Can you work these out from the model? Positions are in its coordinate system, mm. A direction names the side the tool comes from. Give positions to 0.01 mm unless a question says otherwise; leave off trailing zeros. Order: outer loops, then holes, each group sorted by start corner. A loop starts at its lowest first (then second) coordinate and runs counter-clockwise, first axis right, second up. Notation, with made-up numbers: (26, 27) - (55, 27) arc R23 cw to (55, 60) - close; hole circle Ø9 at (53.5, 45.25). An arc over 180 degrees is marked (long way). Answer as a JSON object with one key per item and string values.
```python
from build123d import *

# Parameters (mm, degrees)
F0_W       = 43.8023
F0_H       = 40.5003
F0_R       = 9.72185
F1_DEPTH   = 9.0424
F3_DEPTH   = 25.4
F4_SIZE2   = 2.54
F4_SIZE    = 0.762
F4_2_SIZE2 = 2.54
F4_2_SIZE  = 0.762
F5_R       = 12.65555
F6_DEPTH   = 2.667
F7_R       = 0.254


with BuildPart() as f1:
    # F0 (on Front) → F1 (new body)
    with BuildSketch(Plane.XZ):
        Rectangle(F0_W, F0_H)
        Circle(F0_R, mode=Mode.SUBTRACT)
    extrude(amount=F1_DEPTH)

    # F2 (on Top) → F3 (cut, symmetric)
    with BuildSketch(Plane.XY):
        Polygon((17.653, -6.096), (17.653, -9.144), (17.653, -9.8752817139), (22.691456601, -9.8752817139), (22.691456601, -6.096), align=None)
        Polygon((-17.653, -9.8752817139), (-17.653, -9.144), (-17.653, -6.096), (-22.691456601, -6.096), (-22.691456601, -9.8752817139), align=None)
    extrude(amount=F3_DEPTH, both=True, mode=Mode.SUBTRACT)

    # F4
    f4_edges = [f1.edges().sort_by_distance(p)[0] for p in [
        (-21.90115, 0, 0),
    ]]
    f4_side = f1.faces().sort_by_distance((-21.90115, -3.048, 0))[0]
    chamfer(f4_edges, length=F4_SIZE, length2=F4_SIZE2, reference=f4_side)

    # F4#2
    f4_2_edges = [f1.edges().sort_by_distance(p)[0] for p in [
        (21.90115, 0, 0),
    ]]
    f4_2_side = f1.faces().sort_by_distance((21.90115, -3.048, 0))[0]
    chamfer(f4_2_edges, length=F4_2_SIZE, length2=F4_2_SIZE2, reference=f4_2_side)

    # F5 (on face) → F6 (cut)
    with BuildSketch(Plane(origin=(0, 0, 0), x_dir=(-1, 0, 0), z_dir=(0, 1, 0))):
        Circle(F5_R)
    extrude(amount=-F6_DEPTH, mode=Mode.SUBTRACT)

    # F7
    f7_edges = [f1.edges().sort_by_distance(p)[0] for p in [
        (12.65555, 0, 0),
        (-9.72185, -2.667, 0),
        (0, -9.0424, -20.25015),
        (0, -9.0424, 20.25015),
        (-9.72185, -9.0424, 0),
    ]]
    fillet(f7_edges, radius=F7_R)


solid = f1.part
```
Q1. I'm going to push flat-ended pins straight in: pin 1 Ø2 at (x, z) = (-20, 6.5) entering from -Y; pin 2 Ø17.5 at (x, z) = (0, 0) entering from +Y; pin 3 Ø0.9 at (y, z) = (-8, -2) entering from -X; pin 4 Ø12.5 at (x, z) = (-0.5, -4) entering from +Y. Where does each tip first touch, or does it pass through?
Recorded:
{"pin 1": "stops at y = -6.1", "pin 2": "passes through", "pin 3": "stops at x = -17.65", "pin 4": "stops at y = -2.67"}
Q2. If we section it at C-C, the plane y = -5.25: Please give me the cut outline in (x, z), then the cut area to 3 significant figures.
Recorded:
{"outline": "(-21.9, -20.25) - (21.9, -20.25) - (21.9, 20.25) - (-21.9, 20.25) - close; hole circle Ø19.44 at (0, 0)", "area": "1,480 mm^2"}
Q3. If we section it at D-D, the plane z = 14.5: Please give me the cut outline in (x, y).
Recorded:
{"outline": "(-21.9, -6.1) - (-17.65, -6.1) - (-17.65, -9.04) - (17.65, -9.04) - (17.65, -6.1) - (21.9, -6.1) - (21.9, -0.76) - (19.36, 0) - (-19.36, 0) - (-21.9, -0.76) - close"}
Q4. I need wall thicknesses on L1, parallel to X at y = -4.15, z = 0; L2, parallel to Z at x = 0, y = -6.4; L3, parallel to X at y = -6.2, z = 0. Which ranges of each line are inside material? Lowest first, please.
Recorded:
{"L1": "x = -21.9 to -9.72, 9.72 to 21.9", "L2": "z = -20.25 to -9.72, 9.72 to 20.25", "L3": "x = -17.65 to -9.72, 9.72 to 17.65"}
Q5. We'd pull the mould along X, two halves only. Please class faces 1 (the face through (9.43, -2.667, -3.69)), 2 (the face through (20, -6.096, 0)), 3 (the face through (17.653, -8, 0)), 4 (the face through (-2.11, -5.81, -9.49)): released by +X, released by -X, zero draft, split by the parting line, or undercut.
Recorded:
{"face 1": "undercut", "face 2": "zero draft", "face 3": "released by +X", "face 4": "undercut"}
Q6. Which directions (+Z, -Z, +X, -X, +Y, -Y) give clear straight access to the entire face, cutting with the end or side of a thin tool? Please do faces 5 (the face through (2.743, -1.444, -12.355)), 6 (the face through (-20.613, -0.376, -0.284)), 7 (the face through (-17.653, -8, 0)).
Recorded:
{"face 5": "+Y", "face 6": "+Z, -Z, -X, +Y", "face 7": "+Z, -Z, -X, -Y"}
Q7. If we section it at B-B, the plane x = 0: Please give me the cut outline in (y, z).
Recorded:
{"outline": "(-9.04, -20) arc R0.25 ccw to (-8.79, -20.25) - (0, -20.25) - (0, -12.91) arc R0.25 ccw to (-0.25, -12.66) - (-2.67, -12.66) - (-2.67, -9.98) arc R0.25 ccw to (-2.92, -9.72) - (-8.79, -9.72) arc R0.25 ccw to (-9.04, -9.98) - close; (-9.04, 9.98) arc R0.25 ccw to (-8.79, 9.72) - (-2.92, 9.72) arc R0.25 ccw to (-2.67, 9.98) - (-2.67, 12.66) - (-0.25, 12.66) arc R0.25 ccw to (0, 12.91) - (0, 20.25) - (-8.79, 20.25) arc R0.25 ccw to (-9.04, 20) - close"}
Q8. If we section it at A-A, the plane z = 0: Please give me the cut outline in (x, y).
Recorded:
{"outline": "(-21.9, -6.1) - (-17.65, -6.1) - (-17.65, -9.04) - (-9.98, -9.04) arc R0.25 ccw to (-9.72, -8.79) - (-9.72, -2.92) arc R0.25 ccw to (-9.98, -2.67) - (-12.66, -2.67) - (-12.66, -0.25) arc R0.25 ccw to (-12.91, 0) - (-19.36, 0) - (-21.9, -0.76) - close; (9.72, -8.79) arc R0.25 ccw to (9.98, -9.04) - (17.65, -9.04) - (17.65, -6.1) - (21.9, -6.1) - (21.9, -0.76) - (19.36, 0) - (12.91, 0) arc R0.25 ccw to (12.66, -0.25) - (12.66, -2.67) - (9.98, -2.67) arc R0.25 ccw to (9.72, -2.92) - close"}
